The listing builds one solid part. Answer for the finished solid, in the listing's coordinates (mm). Face numbers are marked on the shaded views. Coordinates: 2 decimals unless noted, no trailing zeros. Loops run counter-clockwise (first coordinate to the right, second up) from the corner with the lowest first, then second, coordinate; pieces in that order, holes last. Notation, with made-up numbers: M -7.75,61 L -3.75,61 A16 cw -3.75,83 Z; hole C 39.25,1.25 d9. An arc over 180 degrees is marked long. Answer as a JSON object with one key per item and string values. Group by question number.
1. A cutting plane is placed at D-D on y = -16. Give the vertices of the cut face in (x, z), and give its area (3 significant figures).
2. A cutting plane is placed at A-A on y = 0. Give the vertices of the cut face in (x, z).
3. Straight lines are drawn through the part: L1, parallel to Y at x = -16, z = 9.35; L2, parallel to X at y = -15.5, z = 8.5; L3, parallel to Y at x = 15, z = 3.75. For each, find the intervals that lie inside material, in ascending order.
4. Given pin 1 (1.9 mm diameter, centred on x = 16, y = 17, fed in from +Z), flat-ended and moving along its own axis, determine where the tip first touches the part or whether it passes through.
5. A cutting plane is placed at C-C on z = 5. Give the vertices of the cut face in (x, y).
6. Determine the mould class of the marked faces 1, 2, 3 and 4 for opening direction X: released by +X, released by -X, zero draft, split by the parting line, or undercut.
from build123d import *

# Parameters (mm, degrees)
SKETCH1_W           = 40
SKETCH1_H           = 40
BOSS_EXTRUDE1_DEPTH = 10
SKETCH2_R           = 19
SKETCH2_R_2         = 1.6
CUT_EXTRUDE1_DEPTH  = 11
FILLET1_R           = 2
SKETCH3_R           = 3.1
CUT_EXTRUDE2_DEPTH  = 3


with BuildPart() as part:
    # Sketch1 → Boss-Extrude1 (new body)
    with BuildSketch(Plane.XY):
        Rectangle(SKETCH1_W, SKETCH1_H)
    extrude(amount=BOSS_EXTRUDE1_DEPTH)

    # Sketch2 → Cut-Extrude1 (cut, through all)
    with BuildSketch(Plane.XY.offset(10)):
        Circle(SKETCH2_R)
        with Locations((-16, 16)):
            Circle(SKETCH2_R_2)
        with Locations((16, 16)):
            Circle(SKETCH2_R_2)
        with Locations((16, -16)):
            Circle(SKETCH2_R_2)
        with Locations((-16, -16)):
            Circle(SKETCH2_R_2)
    extrude(amount=-CUT_EXTRUDE1_DEPTH, mode=Mode.SUBTRACT)

    # Fillet1
    fillet1_edges = [part.edges().sort_by_distance(p)[0] for p in [
        (20, -20, 5),
        (-20, -20, 5),
        (-20, 20, 5),
        (20, 20, 5),
    ]]
    fillet(fillet1_edges, radius=FILLET1_R)

    # Sketch3 → Cut-Extrude2 (cut)
    with BuildSketch(Plane.XY.offset(10)):
        with Locations((-16, -16)):
            Circle(SKETCH3_R)
        with Locations((16, -16)):
            Circle(SKETCH3_R)
        with Locations((16, 16)):
            Circle(SKETCH3_R)
        with Locations((-16, 16)):
            Circle(SKETCH3_R)
    extrude(amount=-CUT_EXTRUDE2_DEPTH, mode=Mode.SUBTRACT)


solid = part.part
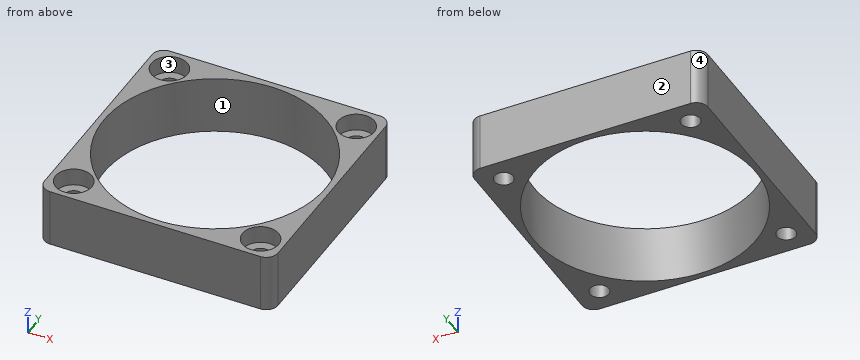
From the geometry:
{
 "1": {"outline": "M -20,0 L -17.6,0 L -17.6,7 L -19.1,7 L -19.1,10 L -20,10 Z; M -14.4,0 L -10.25,0 L -10.25,10 L -12.9,10 L -12.9,7 L -14.4,7 Z; M 10.25,0 L 14.4,0 L 14.4,7 L 12.9,7 L 12.9,10 L 10.25,10 Z; M 17.6,0 L 20,0 L 20,10 L 19.1,10 L 19.1,7 L 17.6,7 Z", "area": "113 mm²"},
 "2": {"outline": "M -20,0 L -19,0 L -19,10 L -20,10 Z; M 19,0 L 20,0 L 20,10 L 19,10 Z"},
 "3": {"L1": "y = -20 to -19.1, -12.9 to -10.25, 10.25 to 12.9, 19.1 to 20", "L2": "x = -20 to -19.06, -12.94 to -10.99, 10.99 to 12.94, 19.06 to 20", "L3": "y = -20 to -17.25, -14.75 to -11.66, 11.66 to 14.75, 17.25 to 20"},
 "4": {"pin 1": "stops at z = 7"},
 "5": {"outline": "M -20,-18 A2 ccw -18,-20 L 18,-20 A2 ccw 20,-18 L 20,18 A2 ccw 18,20 L -18,20 A2 ccw -20,18 Z; hole C 0,0 d38; hole C -16,-16 d3.2; hole C -16,16 d3.2; hole C 16,-16 d3.2; hole C 16,16 d3.2"},
 "6": {"face 1": "undercut", "face 2": "zero draft", "face 3": "undercut", "face 4": "released by -X"}
}
